Here's how the part is built. I have some questions about the finished solid (model axes, mm). Coordinates: 2 decimals unless noted, no trailing zeros. Write each loop counter-clockwise with the first axis right and the second up, starting at its lowest first coordinate (ties: lowest second). Pieces come first, ordered by that corner, then holes. Notation, with made-up numbers: (55.25, -20.75) -> (80.25, -20.75) arc R22 ccw to (80.25, 2.25) -> close; hole circle Ø7 at (23, 22). An arc over 180 degrees is marked (long way). Use CSV: the item, a comma, the result in double quotes. Start each with the question number.
```python
from build123d import *

# Parameters (mm, degrees)
SKETCH1_R           = 37.5
BOSS_EXTRUDE1_DEPTH = 0.8


with BuildPart() as part:
    # Sketch1 → Boss-Extrude1 (new body, symmetric)
    with BuildSketch(Plane(origin=(0, 0, 0), x_dir=(1, 0, 0), z_dir=(0, 1, 0))):
        Circle(SKETCH1_R)
        with BuildLine():
            ThreePointArc((-12.218911, 28.163775), (-12.901924, 28.346788), (-13.084936, 27.663775))
            Line((-13.084936, 27.663775), (-9.001292, 20.590695))
            ThreePointArc((-9.001292, 20.590695), (-7.523035, 19.307531), (-5.568014, 19.2093))
            ThreePointArc((-5.568014, 19.2093), (2.40884, 19.854407), (10, 17.320508))
            ThreePointArc((10, 17.320508), (15.990001, 12.01332), (19.419749, 4.782609))
            ThreePointArc((19.419749, 4.782609), (20.48233, 3.138626), (22.332711, 2.5))
            Line((22.332711, 2.5), (30.5, 2.5))
            ThreePointArc((30.5, 2.5), (31, 3), (30.5, 3.5))
            Line((30.5, 3.5), (22.332711, 3.5))
            ThreePointArc((22.332711, 3.5), (21.099124, 3.925751), (20.390737, 5.021739))
            ThreePointArc((20.390737, 5.021739), (16.789501, 12.613986), (10.5, 18.186533))
            ThreePointArc((10.5, 18.186533), (2.529282, 20.847128), (-5.846415, 20.169765))
            ThreePointArc((-5.846415, 20.169765), (-7.149762, 20.235252), (-8.135267, 21.090695))
            Line((-8.135267, 21.090695), (-12.218911, 28.163775))
        make_face(mode=Mode.SUBTRACT)
        with BuildLine():
            ThreePointArc((10.5, -18.186533), (16.789501, -12.613986), (20.390737, -5.021739))
            ThreePointArc((20.390737, -5.021739), (21.099124, -3.925751), (22.332711, -3.5))
            Line((22.332711, -3.5), (30.5, -3.5))
            ThreePointArc((30.5, -3.5), (31, -3), (30.5, -2.5))
            Line((30.5, -2.5), (22.332711, -2.5))
            ThreePointArc((22.332711, -2.5), (20.48233, -3.138626), (19.419749, -4.782609))
            ThreePointArc((19.419749, -4.782609), (15.990001, -12.01332), (10, -17.320508))
            ThreePointArc((10, -17.320508), (2.40884, -19.854407), (-5.568014, -19.2093))
            ThreePointArc((-5.568014, -19.2093), (-7.523035, -19.307531), (-9.001292, -20.590695))
            Line((-9.001292, -20.590695), (-13.084936, -27.663775))
            ThreePointArc((-13.084936, -27.663775), (-12.901924, -28.346788), (-12.218911, -28.163775))
            Line((-12.218911, -28.163775), (-8.135267, -21.090695))
            ThreePointArc((-8.135267, -21.090695), (-7.149762, -20.235252), (-5.846415, -20.169765))
            ThreePointArc((-5.846415, -20.169765), (2.529282, -20.847128), (10.5, -18.186533))
        make_face(mode=Mode.SUBTRACT)
        with BuildLine():
            ThreePointArc((-21, 0), (-19.318783, -8.233142), (-14.544322, -15.148026))
            ThreePointArc((-14.544322, -15.148026), (-13.949362, -16.309502), (-14.197445, -17.590695))
            Line((-14.197445, -17.590695), (-18.281089, -24.663775))
            ThreePointArc((-18.281089, -24.663775), (-18.098076, -25.346788), (-17.415064, -25.163775))
            Line((-17.415064, -25.163775), (-13.331419, -18.090695))
            ThreePointArc((-13.331419, -18.090695), (-12.959295, -16.168905), (-13.851735, -14.426692))
            ThreePointArc((-13.851735, -14.426692), (-18.398841, -7.841087), (-20, 0))
            ThreePointArc((-20, 0), (-18.398841, 7.841087), (-13.851735, 14.426692))
            ThreePointArc((-13.851735, 14.426692), (-12.959295, 16.168905), (-13.331419, 18.090695))
            Line((-13.331419, 18.090695), (-17.415064, 25.163775))
            ThreePointArc((-17.415064, 25.163775), (-18.098076, 25.346788), (-18.281089, 24.663775))
            Line((-18.281089, 24.663775), (-14.197445, 17.590695))
            ThreePointArc((-14.197445, 17.590695), (-13.949362, 16.309502), (-14.544322, 15.148026))
            ThreePointArc((-14.544322, 15.148026), (-19.318783, 8.233142), (-21, 0))
        make_face(mode=Mode.SUBTRACT)
    extrude(amount=BOSS_EXTRUDE1_DEPTH, both=True)


solid = part.part
```
Item 1: If I drill on line 1 along Z through (x, y) = (-7, -0.4); line 2 along Z through (x, y) = (22, 0.45); line 3 along X through (y, z) = (0, 14.5), over which ranges is the centre line in solid material (lowest first)?
Item 2: I want a section at B-B on z = 13.5. Please give me the cut outline in (x, y).
Item 3: I'm going to push flat-ended pins straight in: pin 1 (0.8 mm diameter, centred on x = 24.5, y = 0, fed in from +Z); pin 2 (0.5 mm diameter, centred on x = 27.5, y = 0, fed in from +Z). Where does each tip first touch, or does it pass through?
Item 4: I want a section at A-A on x = 0. Please give me the cut outline in (y, z).
Item 5: I want a section at D-D on z = 32.5. Please give me the cut outline in (x, y), then the cut area to 3 significant figures.
Item 6: I want a section at C-C on z = -31.5. Please give me the cut outline in (x, y), then the cut area to 3 significant figures.
Geometry says:
1,line 1,"-36.84 to -20.18, -19.15 to 19.15, 20.18 to 36.84"
1,line 2,"-30.37 to -3.53, -2.52 to 2.52, 3.53 to 30.37"
1,line 3,"-34.58 to -15.19, -13.78 to 13.77, 15.19 to 34.58"
2,outline,"(-34.99, -0.8) -> (-16.09, -0.8) -> (-16.09, 0.8) -> (-34.99, 0.8) -> close; (-14.76, -0.8) -> (14.76, -0.8) -> (14.76, 0.8) -> (-14.76, 0.8) -> close; (16.09, -0.8) -> (34.99, -0.8) -> (34.99, 0.8) -> (16.09, 0.8) -> close"
3,pin 1,"z = 28.73"
3,pin 2,"z = 25.76"
4,outline,"(-0.8, -37.5) -> (0.8, -37.5) -> (0.8, -21) -> (-0.8, -21) -> close; (-0.8, -20) -> (0.8, -20) -> (0.8, 20) -> (-0.8, 20) -> close; (-0.8, 21) -> (0.8, 21) -> (0.8, 37.5) -> (-0.8, 37.5) -> close"
5,outline,"(-18.71, -0.8) -> (18.71, -0.8) -> (18.71, 0.8) -> (-18.71, 0.8) -> close"
5,area,"59.9 mm2"
6,outline,"(-20.35, -0.8) -> (20.35, -0.8) -> (20.35, 0.8) -> (-20.35, 0.8) -> close"
6,area,"65.1 mm2"
